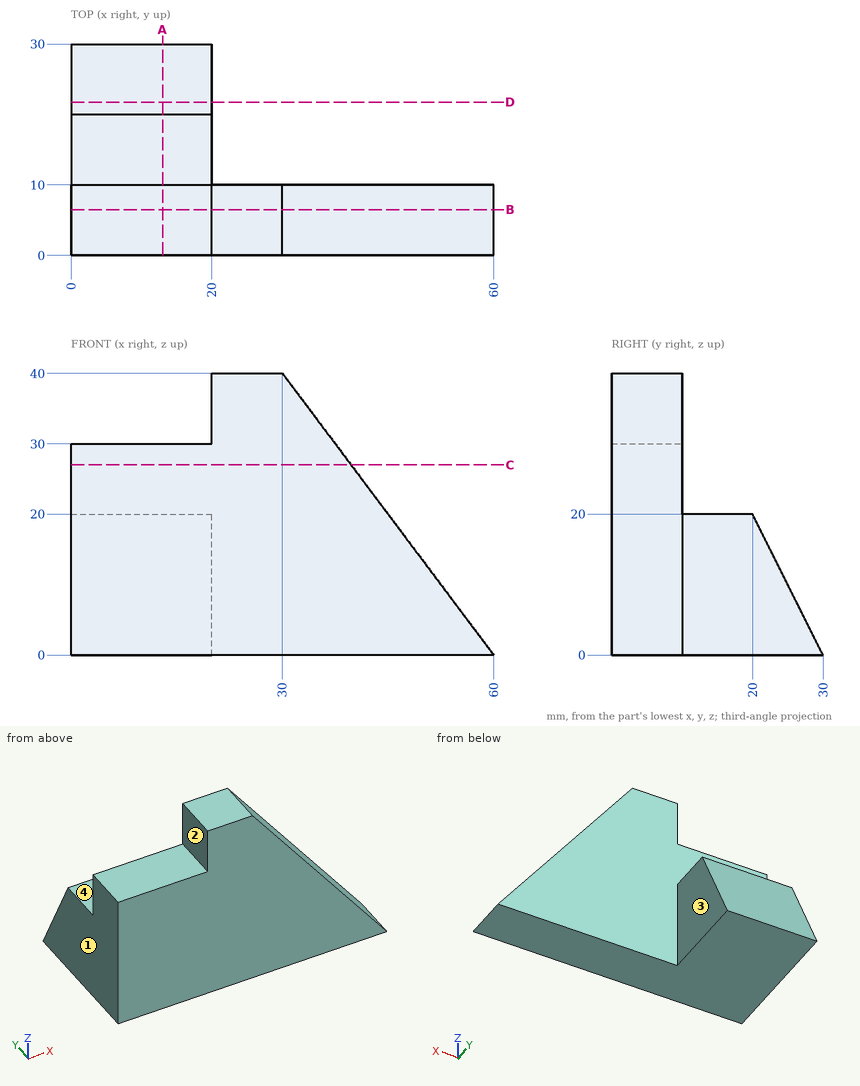
Design review of the part shown in the three views and the two pictorial views. Dimensions are in mm from the part's minimum x, y and z. A direction names the side the tool comes from. Coordinates: 2 decimals unless noted, no trailing zeros. Write each loop counter-clockwise with the first axis right and the second up, starting at its lowest first coordinate (ties: lowest second). Pieces come first, ordered by that corner, then holes.
1) We need section D-D on y = 21.75. State the section outline as (x, z) points, then the cut area to 3 significant figures.
2) Machinability: for the marked faces 1, 2, 3 and 4, which of the approach directions +Z, -Z, +X, -X, +Y, -Y give a long, thin tool a straight path to every point of the face, cutting with its end or side? Answer none if there is none.
3) Clearance check with flat-ended pins moving along their axes: pin 1 Ø11 at (x, y) = (6, 15) entering from +Z; pin 2 Ø10 at (x, y) = (14.5, 24) entering from +Z; pin 3 Ø20 at (x, z) = (39.5, 15.5) entering from +Y. State where each tip first meets the part, or that it passes through.
4) We need section A-A on x = 13. State the section outline as (y, z) points, then the cut area to 3 significant figures.
5) We need section C-C on z = 27. State the section outline as (x, y) points, then the cut area to 4 significant figures.
6) We need section B-B on y = 6.5. State the section outline as (x, z) points, then the cut area to 3 significant figures.
7) To check wall thickness, follow probe 1 along Y at (x, z) = (31, 22); probe 2 along Z at (x, y) = (16, 6); probe 3 along X at (y, z) = (21.5, 4). State the ranges of each line that lie inside material, in increasing order.
Answer list:
1. outline: (0, 0) - (20, 0) - (20, 16.5) - (0, 16.5) - close
1. area: 330 mm2
2. face 1: +Z, -Z, -X, +Y, -Y
2. face 2: +Z, -X, +Y, -Y
2. face 3: +Z, -Z, +X, +Y
2. face 4: +Z, +X, -X, +Y
3. pin 1: stops at z = 30
3. pin 2: stops at z = 20
3. pin 3: stops at y = 10
4. outline: (0, 0) - (30, 0) - (20, 20) - (10, 20) - (10, 30) - (0, 30) - close
4. area: 600 mm2
5. outline: (0, 0) - (39.75, 0) - (39.75, 10) - (0, 10) - close
5. area: 397.5 mm2
6. outline: (0, 0) - (60, 0) - (30, 40) - (20, 40) - (20, 30) - (0, 30) - close
6. area: 1,600 mm2
7. probe 1: y = 0 to 10
7. probe 2: z = 0 to 30
7. probe 3: x = 0 to 20
